Part model, mm, in its own coordinate system. A direction names the side the tool comes from. Give positions to 0.01 mm unless a question says otherwise; leave off trailing zeros. Write each loop counter-clockwise with the first axis right and the second up, starting at its lowest first coordinate (ties: lowest second). Pieces come first, ordered by that corner, then holes.
Autodesk Inventor part; units mm, degrees
ref_plane "YZ Plane" through (0, 0, 0) normal (1, 0, 0) x (0, 1, 0)
ref_plane "XZ Plane" through (0, 0, 0) normal (0, 1, 0) x (-1, 0, 0)
ref_plane "XY Plane" through (0, 0, 0) normal (0, 0, 1) x (1, 0, 0)
sketch "Boceto1" plane through (0, 0, 0) normal (0, 1, 0) x (-1, 0, 0)
  line L0 (50, 10) -> (-50, 10)
  line L1 (-50, 10) -> (-50, -10)
  line L2 (-50, -10) -> (50, -10)
  line L3 (50, -10) -> (50, 10)
  line L4 (50, 10) -> (-50, -10) construction
  line L5 (-50, 10) -> (50, -10) construction
  line L6 (-50, -10) -> (-20, -10)
  line L7 (0, 0) -> (50, 0)
  line L8 (0, 0) -> (0, 10)
  dimension "d0" = 100
  dimension "d1" = 20
  dimension "d2" = 30
extrude "Extrusión1" add sketch "Boceto1" along normal blind 5.5 contours L3 L7 L8 L0
extrude "Extrusión2" add sketch "Boceto1" along normal blind 5.5 contours L8 L7 L3 L2 L1 L0
sketch "Boceto5" plane through (0, 5.5, 0) normal (0, 1, 0) x (1, 0, 0)
  line L0 (50, 10) -> (-50, 10)
  line L1 (20, 0) -> (50, 0)
  circle A0 centre (35, 0) radius 25
  line L2 (35, 25) -> (35, 20)
  line L3 (35, 20) -> (50, 20)
  line L4 (35, 20) -> (20, 20)
  line L5 (35, 0) -> (50, 0)
  point P0 (0, 0)
  point P1 (20, 10)
  dimension "d27" = 50
extrude "Extrusión8" add sketch "Boceto5" against normal blind 5.5
sketch "Boceto6" plane through (0, 5.5, 0) normal (0, 1, 0) x (1, 0, 0)
  line L0 (12.0871, 10) -> (-50, 10)
  line L1 (-50, 10) -> (-50, -10)
  line L2 (-50, -10) -> (12.0871, -10)
  arc A0 (12.0871, -10) -> (12.0871, 10) centre (35, 0) ccw
  line L3 (-50, 10) -> (-50, -10)
  line L4 (-50, 0) -> (-100, 0)
  line L5 (-100, 0) -> (-50, -10)
  line L6 (-100, 0) -> (-100, 50)
  line L7 (-100, 50) -> (-50, 50)
  line L8 (-50, 50) -> (-50, 0)
  line L9 (-100, 25) -> (-50, 25)
  point P0 (0, 0)
  dimension "d33" = 50
  dimension "d34" = 50
extrude "Extrusión9" add sketch "Boceto6" against normal blind 5.5 contours L1 L4 L6 L9 L8 | L1 L5 L4
properties part number "PINZA_I"
1) Saw through at A-A, the plane y = 0.9. Write the cut outline in (x, z).
Answers follow:
outline: (-100, -25) - (-50, -25) - (-50, -10) - (12.09, -10) arc R25 ccw (long way) to (12.09, 10) - (-50, 10) - (-100, 0) - close
2) Two-plate mould, pull along X, no slides. Class faces 4 (the face through (-19, 5.5, -5)), 5 (the face through (59.98, 2.79, 0.96)), 6 (the face through (-75, 3, 5)): +X half, -X half, draft (parallel to the pull), parting line (faces both ways), or undercut.
Answers follow:
face 4: draft
face 5: undercut
face 6: -X half
3) Pin check, flat tip, straight feed: pin 1 Ø3 at (x, y) = (-24.5, 3) entering from -Z. Stop position of the tip, or through.
Answers follow:
pin 1: stops at z = -10
4) Saw through at D-D, the plane z = 2.5. Write the cut outline in (x, y).
Answers follow:
outline: (-87.5, 0) - (59.87, 0) - (59.87, 5.5) - (-87.5, 5.5) - close
5) Saw through at C-C, the plane x = -12. Write the cut outline in (y, z), then the cut area to 3 significant figures.
Answers follow:
outline: (0, -10) - (5.5, -10) - (5.5, 10) - (0, 10) - close
area: 110 mm2
6) Saw through at B-B, the plane z = -13. Write the cut outline in (x, y), then the cut area to 3 significant figures.
Answers follow:
outline: (-100, 0) - (-50, 0) - (-50, 5.5) - (-100, 5.5) - close; (13.65, 0) - (56.35, 0) - (56.35, 5.5) - (13.65, 5.5) - close
area: 510 mm2
7) Wall check: L1, parallel to Z at x = -20.5, y = 3.05; L2, parallel to X at y = 3.2, z = -19.5; L3, parallel to X at y = 1.9, z = -20. Give the ranges that are in metal, low to high.
Answers follow:
L1: z = -10 to 10
L2: x = -100 to -50, 19.36 to 50.64
L3: x = -100 to -50, 20 to 50
8) 3-axis set-ups, long thin cutter, end or side, ignore diameter. For faces 1 (the face through (-19, 3, -10)), 2 (the face through (-100, 3, -12)), 3 (the face through (-19, 3, 10)): which of +Z, -Z, +X, -X, +Y, -Y reach the whole face in a straight line?
Answers follow:
face 1: -Z, +Y, -Y
face 2: +Z, -Z, -X, +Y, -Y
face 3: +Z, -X, +Y, -Y
